```python
from build123d import *

# Parameters (mm, degrees)
F0_W     = 120
F0_H     = 20
F1_DEPTH = 3
F2_R     = 3.1
F3_DEPTH = 25


# Not quite as in the source:
# - a pattern or mirror of a feature is missing from the dataset's text; its kind, count and spacing are read off the source's solid


with BuildPart() as f1:
    # F0 (on Top) → F1 (new body)
    with BuildSketch(Plane.XY):
        Rectangle(F0_W, F0_H)
    extrude(amount=F1_DEPTH)

    # F2 (on face) → F3 (cut)
    with BuildSketch(Plane.XY.offset(3)):
        with Locations((50, 0)):
            Circle(F2_R)
    f3 = extrude(amount=-F3_DEPTH, mode=Mode.SUBTRACT)

    # F3_copies: F3 across plane
    add(f3.mirror(Plane(origin=(0, 0, 0), x_dir=(0, 0, -1), z_dir=(-1, 0, 0))), mode=Mode.SUBTRACT)


solid = f1.part
```
Here's how the part is built. I have some questions about the finished solid (model axes, mm). Coordinates: 2 decimals unless noted, no trailing zeros. Order: outer loops, then holes, each group sorted by start corner. A loop starts at its lowest first (then second) coordinate and runs counter-clockwise, first axis right, second up. Notation, with made-up numbers: (-4, -23.5) -> (35, -23.5) arc R25 cw to (35, 1.5) -> close; hole circle Ø8 at (18, -30.75). An arc over 180 degrees is marked (long way). Return JSON: item names as keys, results as strings.
1) Thinking about a two-plate mould opening in Y: for faces 1 (the flat face through (60, 0, 1)), 2 (the cylindrical face through (-52.864, -1.187, 1.521)), 3 (the flat face through (-1, -10, 1)), which applies, +Y half, -Y half, draft (parallel to the pull), parting line (faces both ways), or undercut?
Conclusion:
{"face 1": "draft", "face 2": "undercut", "face 3": "-Y half"}
2) If we section it at C-C on z = 1.85: List the corners of the cut face in (x, y) for me.
Conclusion:
{"outline": "(-60, -10) -> (60, -10) -> (60, 10) -> (-60, 10) -> close; hole circle Ø6.2 at (-50, 0); hole circle Ø6.2 at (50, 0)"}
3) If we section it at B-B on y = 0: List the corners of the cut face in (x, z) for me.
Conclusion:
{"outline": "(-60, 0) -> (-53.1, 0) -> (-53.1, 3) -> (-60, 3) -> close; (-46.9, 0) -> (46.9, 0) -> (46.9, 3) -> (-46.9, 3) -> close; (53.1, 0) -> (60, 0) -> (60, 3) -> (53.1, 3) -> close"}
4) If I drill on probe 1 along Y at (x, z) = (-50, 2.2); probe 2 along X at (y, z) = (0.5, 2.6); probe 3 along Y at (x, z) = (-48, 2.7), over which ranges is the centre line in solid material (lowest first)?
Conclusion:
{"probe 1": "y = -10 to -3.1, 3.1 to 10", "probe 2": "x = -60 to -53.06, -46.94 to 46.94, 53.06 to 60", "probe 3": "y = -10 to -2.37, 2.37 to 10"}
5) If we section it at A-A on x = 50: List the corners of the cut face in (y, z) for me.
Conclusion:
{"outline": "(-10, 0) -> (-3.1, 0) -> (-3.1, 3) -> (-10, 3) -> close; (3.1, 0) -> (10, 0) -> (10, 3) -> (3.1, 3) -> close"}
